Read the model definition and answer for the solid it produces. Units are mm, in the model's axes. A direction names the side the tool comes from. Coordinates: 2 decimals unless noted, no trailing zeros. Write each loop counter-clockwise with the first axis right and the second up, starting at its lowest first coordinate (ties: lowest second). Pieces come first, ordered by that corner, then holes.
(1) The part is cut by section B-B, the plane y = 21. Determine the outline of the cut face in (x, z).
(2) Given pin 1 (4 mm diameter, centred on x = 40, z = 10.05, fed in from +Y); pin 2 (1.5 mm diameter, centred on x = 46, z = 6.5, fed in from +Y); pin 3 (1.3 mm diameter, centred on y = 22, z = 9, fed in from -X); pin 4 (1.5 mm diameter, centred on y = 20, z = 7, fed in from -X), each flat-ended and moving along its own axis, determine where each tip first touches the part or whether it passes through.
(3) The part is cut by section C-C, the plane z = 16. Determine the outline of the cut face in (x, y), and give its area (3 significant figures).
(4) Which of the six approach directions +Z, -Z, +X, -X, +Y, -Y give full straight-line access (tool end or side, diameter ignored) to faces 1 (the cylindrical face through (58.972, 9.17, 13.413)), 2 (the flat face through (59, 16, 3)), 3 (the flat face through (35, 2, 7.75)), 4 (the cylindrical face through (1.972, 9.17, 13.413)), 5 (the flat face through (2, 18, 10))?
(5) Determine the mould class of faces 6 (the flat face through (36.9, 2.5, 0)), 7 (the flat face through (23, 12.5, 12.4)), 8 (the flat face through (20, 21, 12.25)) for opening direction Z: pulls with the +Z half, pulls with the -Z half, needs draft (parallel to the pull), parting line crosses it, or undercut.
(6) Straight lines are drawn through the part: line 1 along X through (y, z) = (8.5, 13.5); line 2 along X through (y, z) = (16.25, 9.5); line 3 along Y through (x, z) = (3.25, 15). For each, find the intervals that lie inside material, in ascending order.
(7) The part is cut by section D-D, the plane y = 14.25. Determine the outline of the cut face in (x, z).
(8) The part is cut by section A-A, the plane x = 40. Determine the outline of the cut face in (y, z), and give its area (3 significant figures).
```python
from build123d import *

# Parameters (mm, degrees)
SKETCH_1_W          = 80
SKETCH_1_H          = 20
EXTRUDE_1_DEPTH     = 3
SKETCH_2_R          = 3.5
CUT_EXTRUDE_1_DEPTH = 3
SKETCH_3_W          = 15
SKETCH_3_H          = 4.5
CUT_EXTRUDE_2_DEPTH = 2
SKETCH_5_R          = 2.25
CUT_EXTRUDE_3_DEPTH = 2
SKETCH_6_W          = 4
SKETCH_6_H          = 20
EXTRUDE_2_DEPTH     = 15
CUT_EXTRUDE_4_DEPTH = 83
SKETCH_8_R          = 2
CUT_EXTRUDE_5_DEPTH = 83
SKETCH_9_W          = 4
SKETCH_9_H          = 20
EXTRUDE_3_DEPTH     = 25
SKETCH_10_R         = 3.5
CUT_EXTRUDE_6_DEPTH = 6
SKETCH_11_W         = 4.5
SKETCH_11_H         = 15
CUT_EXTRUDE_7_DEPTH = 3
SKETCH_12_R         = 2.25
CUT_EXTRUDE_8_DEPTH = 3


with BuildPart() as part:
    # 草图1 → 凸台-拉伸1 (new body)
    with BuildSketch(Plane(origin=(0, 0, 0), x_dir=(1, 0, 0), z_dir=(0, 1, 0))):
        with Locations((40, -10)):
            Rectangle(SKETCH_1_W, SKETCH_1_H)
    extrude(amount=EXTRUDE_1_DEPTH)

    # 草图2 → 切除-拉伸1 (cut)
    with BuildSketch(Plane(origin=(0, 3, 0), x_dir=(1, 0, 0), z_dir=(0, 1, 0))):
        with Locations(Location((40, -10.045477327, 0), (0, 0, 270))):
            Circle(SKETCH_2_R)
    extrude(amount=-CUT_EXTRUDE_1_DEPTH, mode=Mode.SUBTRACT)

    # 草图3 → 切除-拉伸2 (cut)
    with BuildSketch(Plane(origin=(0, 3, 0), x_dir=(1, 0, 0), z_dir=(0, 1, 0))):
        with Locations((40, -10)):
            Rectangle(SKETCH_3_W, SKETCH_3_H)
    extrude(amount=-CUT_EXTRUDE_2_DEPTH, mode=Mode.SUBTRACT)

    # 草图5 → 切除-拉伸3 (cut)
    with BuildSketch(Plane(origin=(0, 3, 0), x_dir=(1, 0, 0), z_dir=(0, 1, 0))):
        with Locations((32.5, -10)):
            Circle(SKETCH_5_R)
        with Locations((47.5, -10)):
            Circle(SKETCH_5_R)
    extrude(amount=-CUT_EXTRUDE_3_DEPTH, mode=Mode.SUBTRACT)

    # 草图6 → 凸台-拉伸2 (add)
    with BuildSketch(Plane(origin=(0, 3, 0), x_dir=(1, 0, 0), z_dir=(0, 1, 0))):
        with Locations((2, -10)):
            Rectangle(SKETCH_6_W, SKETCH_6_H)
        with Locations((78, -10)):
            Rectangle(SKETCH_6_W, SKETCH_6_H)
        with Locations((59, -10)):
            Rectangle(SKETCH_6_W, SKETCH_6_H)
    extrude(amount=EXTRUDE_2_DEPTH)

    # 草图7 → 切除-拉伸4 (cut)
    with BuildSketch(Plane(origin=(80, 0, 0), x_dir=(0, 0, -1), z_dir=(1, 0, 0))):
        Polygon((-20, 13), (-15, 18), (-20, 18), align=None)
        Polygon((0, 13), (0, 18), (-5, 18), align=None)
    extrude(amount=-CUT_EXTRUDE_4_DEPTH, mode=Mode.SUBTRACT)

    # 草图8 → 切除-拉伸5 (cut)
    with BuildSketch(Plane.ZY):
        with Locations((5, 10.386894075)):
            Circle(SKETCH_8_R)
        with Locations((10, 10.386894075)):
            Circle(SKETCH_8_R)
        with Locations((15, 10.386894075)):
            Circle(SKETCH_8_R)
    extrude(amount=-CUT_EXTRUDE_5_DEPTH, mode=Mode.SUBTRACT)

    # 草图9 → 凸台-拉伸3 (add)
    with BuildSketch(Plane(origin=(0, 3, 0), x_dir=(1, 0, 0), z_dir=(0, 1, 0))):
        with Locations((21, -10)):
            Rectangle(SKETCH_9_W, SKETCH_9_H)
    extrude(amount=EXTRUDE_3_DEPTH)

    # 草图10 → 切除-拉伸6 (cut)
    with BuildSketch(Plane.ZY.offset(-19)):
        with Locations((10, 15.5)):
            Circle(SKETCH_10_R)
    extrude(amount=-CUT_EXTRUDE_6_DEPTH, mode=Mode.SUBTRACT)

    # 草图11 → 切除-拉伸7 (cut)
    with BuildSketch(Plane.ZY.offset(-19)):
        with Locations((10, 15.4)):
            Rectangle(SKETCH_11_W, SKETCH_11_H)
    extrude(amount=-CUT_EXTRUDE_7_DEPTH, mode=Mode.SUBTRACT)

    # 草图12 → 切除-拉伸8 (cut)
    with BuildSketch(Plane.ZY.offset(-19)):
        with Locations((10, 22.9)):
            Circle(SKETCH_12_R)
        with Locations((10, 7.9)):
            Circle(SKETCH_12_R)
    extrude(amount=-CUT_EXTRUDE_8_DEPTH, mode=Mode.SUBTRACT)


solid = part.part
```
Computed:
1. outline: (19, 0) - (23, 0) - (23, 20) - (19, 20) - (19, 12.25) - (22, 12.25) - (22, 7.75) - (19, 7.75) - close
2. pin 1: passes through
2. pin 2: stops at y = 3
2. pin 3: stops at x = 22
2. pin 4: stops at x = 19
3. outline: (0, 0) - (80, 0) - (80, 8.65) - (76, 8.65) - (76, 3) - (61, 3) - (61, 8.65) - (57, 8.65) - (57, 3) - (23, 3) - (23, 28) - (19, 28) - (19, 3) - (4, 3) - (4, 8.65) - (0, 8.65) - close; (0, 12.12) - (4, 12.12) - (4, 17) - (0, 17) - close; (57, 12.12) - (61, 12.12) - (61, 17) - (57, 17) - close; (76, 12.12) - (80, 12.12) - (80, 17) - (76, 17) - close
3. area: 466 mm2
4. face 1: +X
4. face 2: -Z, +X, +Y
4. face 3: +Y
4. face 4: -X
4. face 5: +Z, -Z, -X, +Y
5. face 6: pulls with the -Z half
5. face 7: needs draft
5. face 8: undercut
6. line 1: x = 0 to 4, 19 to 23, 57 to 61, 76 to 80
6. line 2: x = 0 to 4, 57 to 61, 76 to 80
6. line 3: y = 0 to 8.39, 12.39 to 18
7. outline: (0, 1.25) - (4, 1.25) - (4, 18.75) - (0, 18.75) - close; (19, 0) - (23, 0) - (23, 6.73) - (19, 6.73) - close; (19, 13.27) - (23, 13.27) - (23, 20) - (19, 20) - close; (57, 1.25) - (61, 1.25) - (61, 18.75) - (57, 18.75) - close; (76, 1.25) - (80, 1.25) - (80, 18.75) - (76, 18.75) - close
8. outline: (0, 0) - (3, 0) - (3, 6.55) - (0, 6.55) - close; (0, 13.55) - (3, 13.55) - (3, 20) - (0, 20) - close
8. area: 39.0 mm2
